from build123d import *

# Parameters (mm, degrees)
F0_W     = 62
F0_H     = 40.32
F1_DEPTH = 11.5
F2_W     = 25
F2_H     = 9.1
F3_DEPTH = 3.2
F4_W     = 10.9982
F4_H     = 3.114462
F4_H_2   = 3.585538
F5_DEPTH = 1.3
F6_R     = 3.81
F7_R     = 2
F8_DEPTH = 15.24


with BuildPart() as f1:
    # F0 (on Front) → F1 (new body)
    with BuildSketch(Plane.XZ):
        Rectangle(F0_W, F0_H)
    extrude(amount=F1_DEPTH)

    # F2 (on face) → F3 (cut)
    with BuildSketch(Plane.XZ.offset(11.5)):
        Rectangle(F2_W, F2_H)
    extrude(amount=-F3_DEPTH, mode=Mode.SUBTRACT)

    # F4 (on face) → F5 (join)
    with BuildSketch(Plane.XZ.offset(11.5)):
        with Locations((-7.0009, 2.992769)):
            Rectangle(F4_W, F4_H)
        with Locations((-7.0009, -2.757231)):
            Rectangle(F4_W, F4_H_2)
    extrude(amount=-F5_DEPTH)

    # F6
    f6_edges = [f1.edges().sort_by_distance(p)[0] for p in [
        (-31, -5.75, 20.16),
        (31, -5.75, 20.16),
        (31, -5.75, -20.16),
        (-31, -5.75, -20.16),
    ]]
    fillet(f6_edges, radius=F6_R)

    # F7 (on face) → F8 (cut)
    with BuildSketch(Plane.XZ.offset(11.5)):
        with Locations((-24.2824, 0)):
            Circle(F7_R)
        with Locations((24.2824, 0)):
            Circle(F7_R)
    extrude(amount=-F8_DEPTH, mode=Mode.SUBTRACT)


solid = f1.part
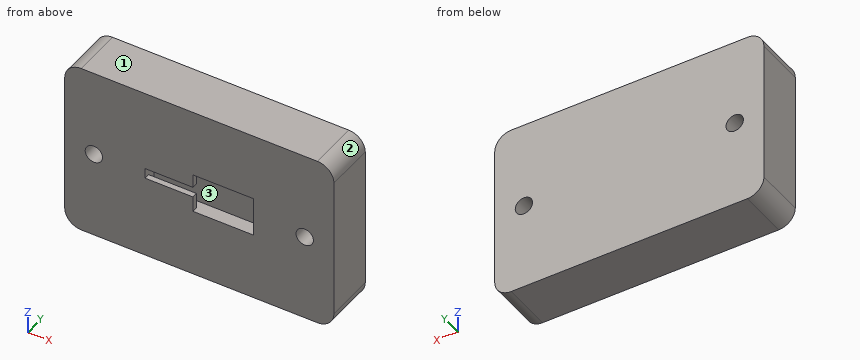
Geometry: final body of the model. Coordinates: model frame, mm. Face numbers are marked on the shaded views. Coordinates: 2 decimals unless noted, no trailing zeros. Order: outer loops, then holes, each group sorted by start corner. A loop starts at its lowest first (then second) coordinate and runs counter-clockwise, first axis right, second up.
1) Draft query along X for the marked faces 1, 2 and 3. Return one class per face: released by +X, released by -X, zero draft, split by the parting line, or undercut.
Result sheet:
face 1: zero draft
face 2: released by +X
face 3: undercut
2) Section B-B (y = -1.5). Return loops of the section in (x, z).
Result sheet:
outline: (-31, -16.35) arc R3.81 ccw to (-27.19, -20.16) - (27.19, -20.16) arc R3.81 ccw to (31, -16.35) - (31, 16.35) arc R3.81 ccw to (27.19, 20.16) - (-27.19, 20.16) arc R3.81 ccw to (-31, 16.35) - close; hole circle Ø4 at (-24.28, 0); hole circle Ø4 at (24.28, 0)
3) Section A-A (z = 0). Return loops of the section in (x, y).
Result sheet:
outline: (-31, -11.5) - (-26.28, -11.5) - (-26.28, 0) - (-31, 0) - close; (-22.28, -11.5) - (-12.5, -11.5) - (-12.5, -8.3) - (12.5, -8.3) - (12.5, -11.5) - (22.28, -11.5) - (22.28, 0) - (-22.28, 0) - close; (26.28, -11.5) - (31, -11.5) - (31, 0) - (26.28, 0) - close
4) Section C-C (x = 25). Return loops of the section in (y, z), then the cut area to 3 significant figures.
Result sheet:
outline: (-11.5, -20.16) - (0, -20.16) - (0, -1.87) - (-11.5, -1.87) - close; (-11.5, 1.87) - (0, 1.87) - (0, 20.16) - (-11.5, 20.16) - close
area: 421 mm2
5) Section D-D (x = -5.5). Return loops of the section in (y, z), then the cut area to 3 significant figures.
Result sheet:
outline: (-11.5, -20.16) - (0, -20.16) - (0, 20.16) - (-11.5, 20.16) - (-11.5, 1.44) - (-10.2, 1.44) - (-10.2, 4.55) - (-8.3, 4.55) - (-8.3, -4.55) - (-10.2, -4.55) - (-10.2, -0.96) - (-11.5, -0.96) - close
area: 443 mm2
6) Ray query, probe 1 along Y at (x, z) = (-7, -3); probe 2 along Y at (x, z) = (8.5, 3); probe 3 along Z at (x, y) = (-11.5, -8.75). Return the intervals inside material, ascending.
Result sheet:
probe 1: y = -11.5 to -10.2, -8.3 to 0
probe 2: y = -8.3 to 0
probe 3: z = -20.16 to -4.55, 4.55 to 20.16
